Read the model definition and answer for the solid it produces. Units are mm, in the model's axes. Give positions to 0.01 mm unless a question says otherwise; leave off trailing zeros. Order: outer loops, then holes, each group sorted by start corner. A loop starts at its lowest first (then second) coordinate and runs counter-clockwise, first axis right, second up.
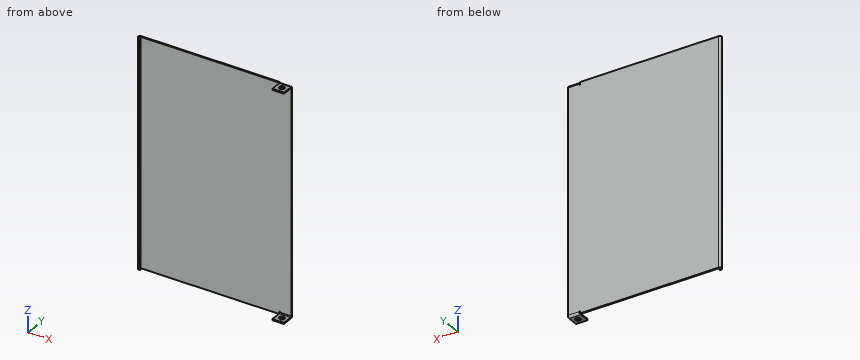
```python
from build123d import *

# Parameters (mm, degrees)
SKETCH1_W                     = 130
SKETCH1_H                     = 194
BASE_FLANGE1_DEPTH            = 1
EDGE_FLANGE1_STRIP_CUT_DEPTH  = 194
EDGE_FLANGE1_DEPTH            = 194
EDGE_FLANGE2_STRIP_W          = 5.4732
EDGE_FLANGE2_STRIP_H          = 1
EDGE_FLANGE2_STRIP_CUT_DEPTH  = 10
EDGE_FLANGE2_RELIEF_W         = 5.9732
EDGE_FLANGE2_RELIEF_H         = 0.5
EDGE_FLANGE2_RELIEF_CUT_DEPTH = 1
EDGE_FLANGE2_DEPTH            = 10
SKETCH14_R                    = 2.25
CUT_EXTRUDE1_DEPTH            = 206.316765339


# Sheet-metal steps are written as plain solids
with BuildPart() as part:
    # Sketch1 → Base-Flange1 (new body)
    with BuildSketch(Plane(origin=(0, 0, 0), x_dir=(1, 0, 0), z_dir=(0, 1, 0))):
        Rectangle(SKETCH1_W, SKETCH1_H)
    extrude(amount=-BASE_FLANGE1_DEPTH)

    # Edge-Flange1 strip (across the edge) → Edge-Flange1 strip cut (cut)
    with BuildSketch(Plane(origin=(-73, -1, 97), x_dir=(0.17364817766693103, 0.984807753012208, 0), z_dir=(0, 0, -1))):
        Polygon((-9.805618071, -61.369193981), (2.446817144, 8.117819101), (1.462009391, 8.291467279), (-10.790425824, -61.195545803), align=None)
    extrude(amount=EDGE_FLANGE1_STRIP_CUT_DEPTH, mode=Mode.SUBTRACT)

    # Edge-Flange1 section (across the edge) → Edge-Flange1 (add)
    with BuildSketch(Plane(origin=(-73, -1, 97), x_dir=(0.17364817766693103, 0.984807753012208, 0), z_dir=(0, 0, -1))):
        with BuildLine():
            Line((-1, 8.419376526), (-1, 9.682776526))
            Line((-1, 9.682776526), (0, 9.682776526))
            Line((0, 9.682776526), (0, 8.419376526))
            ThreePointArc((0, 8.419376526), (0.67240108, 7.685579512), (1.462009391, 8.291467279))
            Line((1.462009391, 8.291467279), (2.446817144, 8.117819101))
            ThreePointArc((2.446817144, 8.117819101), (0.585245337, 6.689384814), (-1, 8.419376526))
        make_face()
    extrude(amount=EDGE_FLANGE1_DEPTH)

    # Edge-Flange2 strip (across the edge) → Edge-Flange2 strip cut (cut)
    with BuildSketch(Plane(origin=(55, -1, -97), x_dir=(0, 0, 1), z_dir=(1, 0, 0))):
        with Locations((-1, -0.5)):
            Rectangle(EDGE_FLANGE2_STRIP_W, EDGE_FLANGE2_STRIP_H)
    edge_flange2_strip_cut = extrude(amount=EDGE_FLANGE2_STRIP_CUT_DEPTH, mode=Mode.SUBTRACT)

    # Edge-Flange2 relief (on the sheet) → Edge-Flange2 relief cut (cut)
    with BuildSketch(Plane(origin=(55, -1, -95.2634), x_dir=(0, 0, 1), z_dir=(0, -1, 0))):
        with Locations((-2.4866, 0.25)):
            Rectangle(EDGE_FLANGE2_RELIEF_W, EDGE_FLANGE2_RELIEF_H)
    edge_flange2_relief_cut = extrude(amount=-EDGE_FLANGE2_RELIEF_CUT_DEPTH, mode=Mode.SUBTRACT)

    # Edge-Flange2 section (across the edge) → Edge-Flange2 (add)
    with BuildSketch(Plane(origin=(55, -1, -97), x_dir=(0, 0, 1), z_dir=(1, 0, 0))):
        with BuildLine():
            Line((0, 0.7366), (0, 10))
            Line((0, 10), (1, 10))
            Line((1, 10), (1, 0.7366))
            ThreePointArc((1, 0.7366), (1.215745145, 0.215745145), (1.7366, 0))
            Line((1.7366, 0), (1.7366, -1))
            ThreePointArc((1.7366, -1), (0.508638364, -0.491361636), (0, 0.7366))
        make_face()
    edge_flange2 = extrude(amount=EDGE_FLANGE2_DEPTH)

    # Sketch14 → Cut-Extrude1 (cut, through all)
    with BuildSketch(Plane(origin=(0, 0, -97), x_dir=(-1, 0, 0), z_dir=(0, 0, -1))):
        with Locations(Location((-60, -6, 0), (0, 0, 90))):
            Circle(SKETCH14_R)
    cut_extrude1 = extrude(amount=-CUT_EXTRUDE1_DEPTH, mode=Mode.SUBTRACT)

    # Mirror1: Edge-Flange2 strip cut, Edge-Flange2 relief cut, Edge-Flange2, Cut-Extrude1 across plane
    add(edge_flange2_strip_cut.mirror(Plane.XY), mode=Mode.SUBTRACT)
    add(edge_flange2_relief_cut.mirror(Plane.XY), mode=Mode.SUBTRACT)
    add(edge_flange2.mirror(Plane.XY))
    add(cut_extrude1.mirror(Plane.XY), mode=Mode.SUBTRACT)


solid = part.part
```
1) The part is cut by section B-B on y = -6. Determine the outline of the cut face in (x, z), and give its area (3 significant figures).
Final values:
outline: (55, -97) - (57.75, -97) - (57.75, -96) - (55, -96) - close; (55, 96) - (57.75, 96) - (57.75, 97) - (55, 97) - close; (62.25, -97) - (65, -97) - (65, -96) - (62.25, -96) - close; (62.25, 96) - (65, 96) - (65, 97) - (62.25, 97) - close
area: 11.0 mm2
2) Given pin 1 (12 mm diameter, centred on x = -39, z = -63, fed in from -Y); pin 2 (1.8 mm diameter, centred on y = -5.5, z = -95.5, fed in from -X), each flat-ended and moving along its own axis, determine where each tip first touches the part or whether it passes through.
Final values:
pin 1: stops at y = -1
pin 2: stops at x = 55
3) The part is cut by section A-A on x = 60. Determine the outline of the cut face in (y, z).
Final values:
outline: (-11, -97) - (-8.25, -97) - (-8.25, -96) - (-11, -96) - close; (-11, 96) - (-8.25, 96) - (-8.25, 97) - (-11, 97) - close; (-3.75, -97) - (-1.74, -97) arc R1.74 ccw to (0, -95.26) - (0, 95.26) arc R1.74 ccw to (-1.74, 97) - (-3.75, 97) - (-3.75, 96) - (-1.74, 96) arc R0.74 cw to (-1, 95.26) - (-1, -95.26) arc R0.74 cw to (-1.74, -96) - (-3.75, -96) - close
4) The part is cut by section C-C on z = -65. Determine the outline of the cut face in (x, y), and give its area (3 significant figures).
Final values:
outline: (-64.88, -3.45) - (-63.64, -3.67) - (-63.46, -2.68) - (-64.71, -2.46) arc R0.74 cw to (-64.58, -1) - (65, -1) - (65, 0) - (-64.58, 0) arc R1.74 ccw to start
area: 135 mm2
5) The part is cut by section D-D on x = 30. Determine the outline of the cut face in (y, z), and give its area (3 significant figures).
Final values:
outline: (-1, -97) - (0, -97) - (0, 97) - (-1, 97) - close
area: 194 mm2
6) Consider L1, parallel to X at y = -6, z = 96.3; L2, parallel to Y at x = 45.5, z = 51.5; L3, parallel to Y at x = 60, z = 96.25. Determine where each line is inside the solid, lowest interval first.
Final values:
L1: x = 55 to 57.75, 62.25 to 65
L2: y = -1 to 0
L3: y = -11 to -8.25, -3.75 to -0.31
